The listing builds one solid part. Answer for the finished solid, in the listing's coordinates (mm). Face numbers are marked on the shaded views. A direction names the side the tool comes from. Round coordinates to 2 decimals unless told otherwise and drop trailing zeros. Order: outer loops, then holes, each group sorted by start corner. A loop starts at its lowest first (then second) coordinate and runs counter-clockwise, first axis right, second up. Notation, with made-up numbers: M 6,56.25 L 18,56.25 A23 ccw 18,65.25 Z; hole C -15,-16 d1. An arc over 180 degrees is marked long. Write item = value, one per line. Start each with the question number.
(1) Straight lines are drawn through the part: probe 1 along Y at (x, z) = (45, 92); probe 2 along Z at (x, y) = (24, 284.5). For each, find the intervals that lie inside material, in ascending order. Write a range as from..to.
(2) A cutting plane is placed at A-A, the plane z = 101. Determine the outline of the cut face in (x, y), and give its area (3 significant figures).
(3) Each of these flat-tipped pins is pushed along its axis until it touches: pin 1 (12 mm diameter, centred on x = 28.5, y = 375, fed in from +Z); pin 2 (21.5 mm diameter, centred on x = 33.5, z = 102.5, fed in from +Y); pin 3 (21.5 mm diameter, centred on x = -3, z = 94, fed in from -Y). Where does it stop, or does it pass through?
(4) Which of the six approach directions +Z, -Z, +X, -X, +Y, -Y give full straight-line access (tool end or side, diameter ignored) to the marked faces 1, 2, 3 and 4?
(5) A cutting plane is placed at B-B, the plane x = 15. Determine the outline of the cut face in (y, z), and give its area (3 significant figures).
(6) A cutting plane is placed at C-C, the plane y = 286. Determine the outline of the cut face in (x, z).
from build123d import *

# Parameters (mm, degrees)
SKETCH1_W           = 100
SKETCH1_H           = 100
BOSS_EXTRUDE1_DEPTH = 500
SKETCH2_W           = 100
SKETCH2_H           = 50
BOSS_EXTRUDE2_DEPTH = 43


with BuildPart() as part:
    # Sketch1 → Boss-Extrude1 (new body)
    with BuildSketch(Plane(origin=(0, 0, 0), x_dir=(1, 0, 0), z_dir=(0, 1, 0))):
        with Locations((19.377593361, -29.709543568)):
            Rectangle(SKETCH1_W, SKETCH1_H)
    extrude(amount=BOSS_EXTRUDE1_DEPTH)

    # Sketch2 → Boss-Extrude2 (add)
    with BuildSketch(Plane.XY.offset(79.709543568)):
        with Locations((19.377593361, 412.588238816)):
            Rectangle(SKETCH2_W, SKETCH2_H)
        with Locations((19.377593361, 162.588238816)):
            Rectangle(SKETCH2_W, SKETCH2_H)
    extrude(amount=BOSS_EXTRUDE2_DEPTH)


solid = part.part
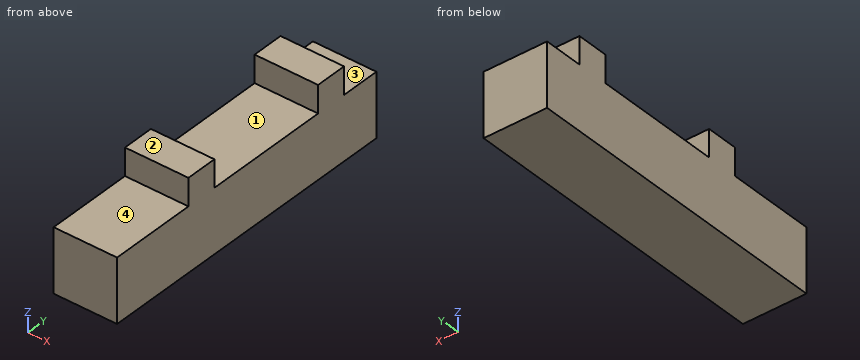
Reported:
q1.probe_1 = 137.59..187.59, 387.59..437.59
q1.probe_2 = -20.29..79.71
q2.outline = M -30.62,137.59 L 69.38,137.59 L 69.38,187.59 L -30.62,187.59 Z; M -30.62,387.59 L 69.38,387.59 L 69.38,437.59 L -30.62,437.59 Z
q2.area = 10,000 mm²
q3.pin_1 = 79.71
q3.pin_2 = 437.59
q3.pin_3 = 137.59
q4.face_1 = +Z, +X, -X
q4.face_2 = +Z, +X, -X, +Y, -Y
q4.face_3 = +Z, +X, -X, +Y
q4.face_4 = +Z, +X, -X, -Y
q5.outline = M 0,-20.29 L 500,-20.29 L 500,79.71 L 437.59,79.71 L 437.59,122.71 L 387.59,122.71 L 387.59,79.71 L 187.59,79.71 L 187.59,122.71 L 137.59,122.71 L 137.59,79.71 L 0,79.71 Z
q5.area = 54,300 mm²
q6.outline = M -30.62,-20.29 L 69.38,-20.29 L 69.38,79.71 L -30.62,79.71 Z
